Autodesk Inventor part; units mm, degrees
ref_plane "Konstruktionshilfsebene" through (0, 0, 0) normal (0, -1, 0) x (1, 0, 0)
ref_plane "Konstruktionshilfsebene:2" through (0, 0, 10) normal (0, 0, -1) x (-1, 0, 0)
ref_plane "YZ Plane" through (0, 0, 0) normal (1, 0, 0) x (0, 1, 0)
sketch "Skizze1" plane through (0, 0, 0) normal (0, 0, 1) x (1, 0, 0)
  arc A0 (30, 0) -> (-30, 0) centre (0, 0) ccw
  line L0 (-17, -35) -> (-17, -55)
  line L1 (-17, -55) -> (-30, -55)
  line L2 (-30, -55) -> (-30, 0)
  line L3 (0, 0) -> (0, 30) construction
  line L4 (17, -35) -> (17, -55)
  line L5 (17, -55) -> (30, -55)
  line L6 (30, -55) -> (30, 0)
  line L7 (-17, -35) -> (17, -35)
  dimension "SJ_D_out" = 60
  dimension "d1" = 55
  dimension "d2" = 17
  dimension "d3" = 35
  dimension "d34" = 13
extrude "Grundform" add sketch "Skizze1" along normal blind 20
fillet "Konturverrundungen" radius 10 4 edges at (-23.5, -55, 20) (23.5, -55, 20) (-23.5, -55, 0) (23.5, -55, 0)
fillet "Konturverrundungen" radius 3 2 edges at (-17, -35, 10) (17, -35, 10)
ref_plane "Konstruktionshilfsebene" through (0, 0, 0) normal (0, -1, 0) x (1, 0, 0)
ref_plane "Arbeitsebene1" through (0, 30, 0) normal (0, -1, 0) x (1, 0, 0)
sketch "Skizze2" plane through (0, 0, 0) normal (0, -1, 0) x (1, 0, 0)
  line L0 (-30, 0) -> (-17, 0) construction
  line L1 (-18, 0) -> (-18, 10)
  line L2 (-17, 20) -> (-17, 0) construction
  line L3 (-18, 10) -> (0, 10)
  line L4 (0, 10) -> (0, 0)
  line L5 (-17, 0) -> (-14, 0) construction
  line L6 (-18, 0) -> (0, 0)
  dimension "d11" = 36
  dimension "d12" = 10
revolve "Wellenaufnahme" cut sketch "Skizze2" angle 360 about axis through (0, 0, 10) along (0, 0, -1)
sketch "Skizze3" plane through (0, 0, 20) normal (0, 0, 1) x (1, 0, 0)
  point P0 (0, 0)
  point P1 (0, 0)
hole "Senkung für M8 Innensechskantschraube" at (0, 0, 20) direction (0, 0, -1) diameter 8.4 end through all countersink diameter 19 countersink angle 90
ref_plane "Konstruktionshilfsebene:2" through (0, 0, 10) normal (0, 0, -1) x (-1, 0, 0)
sketch "Skizze4" plane through (0, 0, 10) normal (0, 0, -1) x (-1, 0, 0)
  line L0 (-30, -45) -> (-30, 0) construction
  line L1 (-17, -38.5) -> (-17, -45)
  line L2 (-30, -45) -> (-17, -45)
  line L3 (-17, -45) -> (-30, -45)
  line L4 (-30, -45) -> (-30, -37.5)
  line L5 (0, 0) -> (0, -35) construction
  line L6 (14, -35) -> (-14, -35) construction
  line L7 (-17, -38) -> (-17, -45) construction
  line L8 (42, -45) -> (-42, -45) construction
  line L9 (-30, -37.5) -> (-22, -37.5)
  line L10 (-22, -37.5) -> (-22, -38.5)
  line L11 (-22, -38.5) -> (-17, -38.5)
  line L12 (17, -38.5) -> (17, -45)
  line L13 (30, -45) -> (17, -45)
  line L14 (17, -45) -> (30, -45)
  line L15 (30, -45) -> (30, -37.5)
  line L16 (30, -37.5) -> (22, -37.5)
  line L17 (22, -37.5) -> (22, -38.5)
  line L18 (22, -38.5) -> (17, -38.5)
  dimension "d35" = 13
  dimension "d39" = 15
  dimension "d40" = 8
revolve "Axial-Radial Nadellager Innenprofil" cut sketch "Skizze4" angle 360 about axis through (8.5, -45, 10) along (1, 0, 0)
sketch "Skizze5" plane through (30, 0, 20) normal (1, 0, 0) x (0, 0, -1)
  circle A0 centre (5, -30.5) radius 1.2 construction
  circle A1 centre (15, -30.5) radius 1.2 construction
  point P0 (20, 0)
hole "Gewinde_Keine_ISO Metrisches Profil_2_Winkel(2)" at (30, -30.5, 15) at (30, -30.5, 5) direction (-1, 0, 0) diameter 1.567 depth 10 tip angle 118
ref_plane "Spiegelebene" through (0, 0, 20) normal (1, 0, 0) x (0, 0, -1)
mirror "Gewindebohrung gespiegelt" about plane through (0, 0, 20) normal (1, 0, 0) of "Gewinde_Keine_ISO Metrisches Profil_2_Winkel(2)"
chamfer "Ansenkung Gewindebohrung M2x0,4mm" distance 0.4 angle 45 4 edges at (30, -30.5, 15.7835) (30, -30.5, 5.7835) (-30, -30.5, 15.7835) (-30, -30.5, 5.7835)
sketch "Sketch6" plane through (0, 0, 20) normal (0, 0, 1) x (1, 0, 0)
  circle A0 centre (0, 0) radius 4.2 construction
  circle A1 centre (0, 0) radius 23.75 construction
  circle A2 centre (0, 0) radius 9.5 construction
  line L0 (0, 0) -> (0, 23.75) construction
  line L1 (23.75, 0) -> (-23.75, 0) construction
  line L2 (0, 0) -> (23.75, 0) construction
  dimension "FixHole_Rad" = 23.75
  dimension "FixHole_Side_Angle" = 90
hole "Hole3" at (0, 23.75, 20) at (-23.75, 0, 20) at (23.75, 0, 20) direction (0, 0, -1) diameter 3.242 depth 12 tip angle 118
chamfer "Chamfer2" distance 0.7 angle 45 3 edges at (-23.75, 1.621, 20) (23.75, 1.621, 20) (0, 25.371, 20)
ref_plane "Arbeitsebene5" through (0, 0, 20) normal (1, 0, 0) x (0, 0, -1)
equation "\"d6\" = 0.5 * d4"
properties part number "Shoulder_Joint_v2" material "PVC-Piping"
Model file for the job. Use its own axes, mm. A direction names the side the tool comes from. Give positions to 0.01 mm unless a question says otherwise; leave off trailing zeros. Order: outer loops, then holes, each group sorted by start corner. A loop starts at its lowest first (then second) coordinate and runs counter-clockwise, first axis right, second up. Notation, with made-up numbers: (-15.75, -34.75) - (27.25, -34.75) arc R21 ccw to (27.25, -29.75) - close; hole circle Ø4 at (85.5, 48). An arc over 180 degrees is marked (long way). One line per item, written item: value.
Item 1: Slice it at B-B (x = 15.5). List the corners of the cut face in (y, z).
Response values:
outline: (-35.4, 0) - (-9.15, 0) - (-9.15, 10) - (9.15, 10) - (9.15, 0) - (25.69, 0) - (25.69, 20) - (-35.4, 20) - close
Item 2: Wall check: line 1 (Z direction, x = -19, y = -45); line 2 (Z direction, x = -23, y = -31); line 3 (Y direction, x = -23.75, z = 12.25). Give the ranges that are in metal, low to high.
Response values:
line 1: 0 to 3.5, 16.5 to 20
line 2: 0 to 4.4, 5.6 to 14.4, 15.6 to 20
line 3: -54.74 to -52.15, -37.85 to -1.62, 1.62 to 18.33
Item 3: Tool access for faces 4 (the cylindrical face through (16.14, -35.9, 10.14)), 5 (the cylindrical face through (-25.944, -41.539, 3.346)), 6 (the cylindrical face through (25.332, 0.351, 13.571)): list every direction of +Z, -Z, +X, -X, +Y, -Y with a clear straight run to the whole face (end or side of a thin tool).
Response values:
face 4: +Z, -Z, -Y
face 5: -X
face 6: +Z
Item 4: Two-plate mould, pull along X, no slides. Class faces 1 (the flat face through (0, -35, 10)), 2 (the flat face through (-30, -22, 10)), 3 (the cylindrical face through (-23.59, -51.99, 2.85)): released by +X, released by -X, zero draft, split by the parting line, or undercut.
Response values:
face 1: undercut
face 2: released by -X
face 3: zero draft
Item 5: Pin check, flat tips, straight feed: pin 1 Ø6 at (x, z) = (-5, 7) entering from -Y; pin 2 Ø0.9 at (y, z) = (-30.5, 15) entering from -X; pin 3 Ø1.4 at (y, z) = (-30.5, 5) entering from +X; pin 4 Ø12 at (y, z) = (-45, 10) entering from +X. Stop position of each tip, or through.
Response values:
pin 1: y = -35
pin 2: x = -19.8
pin 3: x = 19.95
pin 4: through
Item 6: Slice it at A-A (z = 11). Give the number of separate pieces and of enclosed holes in the cut face, then the cut area to 3 significant figures.
Response values:
separate pieces: 3
enclosed holes: 4
area: 3,590 mm2
